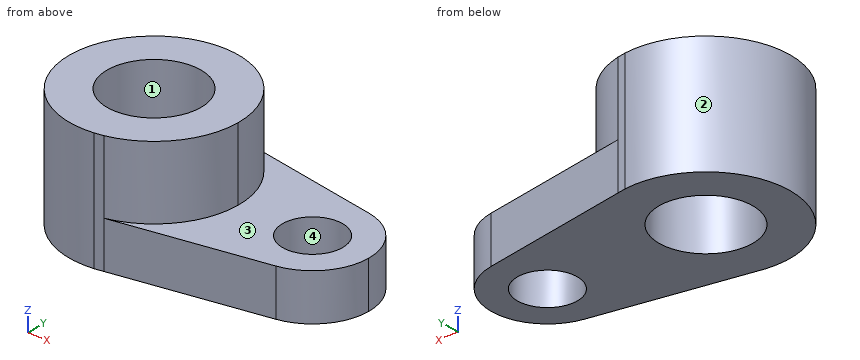
from build123d import *

# Parameters (mm, degrees)
F0_R     = 15.875
F0_R_2   = 10.16
F1_DEPTH = 15.7734
F2_R     = 15.875
F3_DEPTH = 24.4602


with BuildPart() as f1:
    # F0 (on Top) → F1 (new body)
    with BuildSketch(Plane.XY):
        with BuildLine():
            Line((6.4681247744, 27.833325114), (3.5634199556, 28.3519428474))
            ThreePointArc((3.5634199556, 28.3519428474), (-28.575, 0), (3.5634199556, -28.3519428474))
            Line((3.5634199556, -28.3519428474), (6.4681247744, -27.833325114))
            ThreePointArc((6.4681247744, -27.833325114), (22.3758495976, -17.7722249532), (28.575, 0))
            ThreePointArc((28.575, 0), (22.3758495976, 17.7722249532), (6.4681247744, 27.833325114))
        make_face()
        Circle(F0_R, mode=Mode.SUBTRACT)
        with BuildLine():
            Line((57.3233139044, 18.7534341921), (6.4681247744, 27.833325114))
            ThreePointArc((6.4681247744, 27.833325114), (22.3758495976, 17.7722249532), (28.575, 0))
            ThreePointArc((28.575, 0), (22.3758495976, -17.7722249532), (6.4681247744, -27.833325114))
            Line((6.4681247744, -27.833325114), (57.3233139044, -18.7534341921))
            ThreePointArc((57.3233139044, -18.7534341921), (34.925, 0), (57.3233139044, 18.7534341921))
        make_face()
        with BuildLine():
            ThreePointArc((73.025, 0), (68.5812979546, 12.2294137251), (57.3233139044, 18.7534341921))
            ThreePointArc((57.3233139044, 18.7534341921), (34.925, 0), (57.3233139044, -18.7534341921))
            ThreePointArc((57.3233139044, -18.7534341921), (68.5812979546, -12.2294137251), (73.025, 0))
        make_face()
        with Locations((53.975, 0)):
            Circle(F0_R_2, mode=Mode.SUBTRACT)
    extrude(amount=F1_DEPTH)

    # F2 (on face) → F3 (join)
    with BuildSketch(Plane.XY.offset(15.7734)):
        with BuildLine():
            Line((6.4681247744, 27.833325114), (3.5634199556, 28.3519428474))
            ThreePointArc((3.5634199556, 28.3519428474), (-28.575, 0), (3.5634199556, -28.3519428474))
            Line((3.5634199556, -28.3519428474), (6.4681247744, -27.833325114))
            ThreePointArc((6.4681247744, -27.833325114), (22.3758495976, -17.7722249532), (28.575, 0))
            ThreePointArc((28.575, 0), (22.3758495976, 17.7722249532), (6.4681247744, 27.833325114))
        make_face()
        Circle(F2_R, mode=Mode.SUBTRACT)
    extrude(amount=F3_DEPTH)


solid = f1.part
Could you check a few things on this model? Use its own coordinates, in mm. Face numbers are marked on the shaded views. Coordinates: 2 decimals unless noted, no trailing zeros. Order: outer loops, then holes, each group sorted by start corner. A loop starts at its lowest first (then second) coordinate and runs counter-clockwise, first axis right, second up. Notation, with made-up numbers: (63.5, -33.75) -> (85.5, -33.75) arc R23 ccw to (85.5, -4.75) -> close; hole circle Ø3 at (8.25, 48.5). An arc over 180 degrees is marked (long way). One line per question, with ' | ' between items.
Q1. I'm going to push flat-ended pins straight in: P1, Ø3, axis at y = -20.5, z = 17, coming from the -X side; P2, Ø5, axis at y = -5, z = 35, coming from the +X side; P3, Ø4, axis at x = -4, z = 17, coming from the -Y side; P4, Ø2, axis at x = 59, y = -21, coming from the +Z side. Where does each tip first touch, or does it pass through?
Return value:
P1: x = -21.34 | P2: x = 28.47 | P3: y = -28.5 | P4: through
Q2. Imagine slicing it at A-A on x = 0. Please give me the cut outline in (y, z) (3 decimals), and give its area (3 significant figures).
Return value:
outline: (-28.575, 0) -> (-15.875, 0) -> (-15.875, 40.234) -> (-28.575, 40.234) -> close; (15.875, 0) -> (28.575, 0) -> (28.575, 40.234) -> (15.875, 40.234) -> close | area: 1,020 mm²
Q3. Thinking about a two-plate mould opening in Y: for the marked faces 1, 2, 3 and 4, which applies, pulls with the +Y half, pulls with the -Y half, needs draft (parallel to the pull), parting line crosses it, or undercut?
Return value:
face 1: undercut | face 2: parting line crosses it | face 3: needs draft | face 4: undercut
Q4. If I drill on L1, parallel to Y at x = 0, z = 28 (3 decimals); L2, parallel to X at y = 7, z = 7.5; L3, parallel to Y at x = 12, z = 16, over which ranges is the centre line in solid material (lowest first)?
Return value:
L1: -28.575 to -15.875, 15.875 to 28.575 | L2: -27.7 to -14.25, 14.25 to 46.61, 61.34 to 71.69 | L3: -25.93 to -10.39, 10.39 to 25.93
Q5. Imagine slicing it at C-C on y = -5.5. Please give me the cut outline in (x, z), and give its area (3 significant figures).
Return value:
outline: (-28.04, 0) -> (-14.89, 0) -> (-14.89, 40.23) -> (-28.04, 40.23) -> close; (14.89, 0) -> (45.43, 0) -> (45.43, 15.77) -> (28.04, 15.77) -> (28.04, 40.23) -> (14.89, 40.23) -> close; (62.52, 0) -> (72.21, 0) -> (72.21, 15.77) -> (62.52, 15.77) -> close | area: 1,490 mm²
Q6. Imagine slicing it at D-D on y = -14. Please give me the cut outline in (x, z).
Return value:
outline: (-24.91, 0) -> (-7.48, 0) -> (-7.48, 40.23) -> (-24.91, 40.23) -> close; (7.48, 0) -> (66.89, 0) -> (66.89, 15.77) -> (24.91, 15.77) -> (24.91, 40.23) -> (7.48, 40.23) -> close
Q7. Imagine slicing it at B-B on z = 18. Please give me the cut outline in (x, y) (3 decimals).
Return value:
outline: (3.563, -28.352) -> (6.468, -27.833) arc R28.575 ccw to (6.468, 27.833) -> (3.563, 28.352) arc R28.575 ccw (long way) to start; hole circle Ø31.75 at (0, 0)
